Input: part model. Units: mm. Frame: model coordinates. A direction names the side the tool comes from. Give positions to 0.01 mm unless a question says otherwise; leave off trailing zeros. Loops run counter-clockwise (first coordinate to the right, second up) from the corner with the lowest first, then second, coordinate; pieces in that order, holes last.
from build123d import *

# Parameters (mm, degrees)
SKETCH_1_W          = 45.22
SKETCH_1_H          = 24.72
SKETCH_1_R          = 9.6
SKETCH_1_R_2        = 1
EXTRUDE_1_DEPTH     = 3
SKETCH_2_W          = 3
SKETCH_2_H          = 24.72
EXTRUDE_2_DEPTH     = 10
SKETCH_3_W          = 24.72
SKETCH_3_H          = 3
EXTRUDE_3_DEPTH     = 45.22
SKETCH_4_R          = 9.6
SKETCH_4_R_2        = 1
CUT_EXTRUDE_1_DEPTH = 4
FILLET_3_R          = 10
FILLET_4_R          = 5
FILLET_5_R          = 5
FILLET_6_R          = 5
FILLET_7_R          = 5


with BuildPart() as part:
    # 草图1 → 凸台-拉伸1 (new body)
    with BuildSketch(Plane.XY):
        with Locations((21.400674487, -11.617565982)):
            Rectangle(SKETCH_1_W, SKETCH_1_H)
        with Locations((33.900674487, -11.617565982)):
            Circle(SKETCH_1_R, mode=Mode.SUBTRACT)
        with Locations((25.600674487, -1.257565982)):
            Circle(SKETCH_1_R_2, mode=Mode.SUBTRACT)
        with Locations((4.900674487, -1.257565982)):
            Circle(SKETCH_1_R_2, mode=Mode.SUBTRACT)
        with Locations((4.900674487, -21.977565982)):
            Circle(SKETCH_1_R_2, mode=Mode.SUBTRACT)
        with Locations((25.600674487, -21.977565982)):
            Circle(SKETCH_1_R_2, mode=Mode.SUBTRACT)
    extrude(amount=EXTRUDE_1_DEPTH)

    # 草图2 → 凸台-拉伸2 (add)
    with BuildSketch(Plane.ZY.offset(1.209325513)):
        with Locations((1.5, -11.617565982)):
            Rectangle(SKETCH_2_W, SKETCH_2_H)
    extrude(amount=EXTRUDE_2_DEPTH)

    # 草图3 → 凸台-拉伸3 (add)
    with BuildSketch(Plane(origin=(0, 0.742434018, 0), x_dir=(1, 0, 0), z_dir=(0, 1, 0))):
        with Locations((1.150674487, -1.5)):
            Rectangle(SKETCH_3_W, SKETCH_3_H)
    extrude(amount=EXTRUDE_3_DEPTH)

    # 草图4 → 切除-拉伸1 (cut)
    with BuildSketch(Plane.XY.offset(3)):
        with Locations((1.150674487, 35.852434018)):
            Circle(SKETCH_4_R)
        with Locations((-9.209325513, 27.552434018)):
            Circle(SKETCH_4_R_2)
        with Locations((11.510674487, 27.552434018)):
            Circle(SKETCH_4_R_2)
        with Locations((11.510674487, 6.852434018)):
            Circle(SKETCH_4_R_2)
        with Locations((-9.209325513, 6.852434018)):
            Circle(SKETCH_4_R_2)
    extrude(amount=-CUT_EXTRUDE_1_DEPTH, mode=Mode.SUBTRACT)

    # 圆角3
    fillet_3_edges = [part.edges().sort_by_distance(p)[0] for p in [
        (-11.209325513, -23.977565982, 1.5),
    ]]
    fillet(fillet_3_edges, radius=FILLET_3_R)

    # 圆角4
    fillet_4_edges = [part.edges().sort_by_distance(p)[0] for p in [
        (44.010674487, -23.977565982, 1.5),
    ]]
    fillet(fillet_4_edges, radius=FILLET_4_R)

    # 圆角5
    fillet_5_edges = [part.edges().sort_by_distance(p)[0] for p in [
        (44.010674487, 0.742434018, 1.5),
    ]]
    fillet(fillet_5_edges, radius=FILLET_5_R)

    # 圆角6
    fillet_6_edges = [part.edges().sort_by_distance(p)[0] for p in [
        (-11.209325513, 45.962434018, 1.5),
    ]]
    fillet(fillet_6_edges, radius=FILLET_6_R)

    # 圆角7
    fillet_7_edges = [part.edges().sort_by_distance(p)[0] for p in [
        (13.510674487, 45.962434018, 1.5),
    ]]
    fillet(fillet_7_edges, radius=FILLET_7_R)


solid = part.part
(1) Cut plane A-A (y = -17). Return the cut outline in (x, z), and give its area (3 significant figures).
Values follow:
outline: (-10.74, 0) - (25.95, 0) - (25.95, 3) - (-10.74, 3) - close; (41.85, 0) - (44.01, 0) - (44.01, 3) - (41.85, 3) - close
area: 117 mm2
(2) Ray query, probe 1 along Y at (x, z) = (11, 1.4); probe 2 along X at (y, z) = (28, 0.6); probe 3 along Y at (x, z) = (5, 1.45). Return the intervals inside material, ascending.
Values follow:
probe 1: y = -23.98 to 5.99, 7.71 to 26.69, 28.41 to 45.3
probe 2: x = -11.21 to -10.1, -8.32 to -4.37, 6.67 to 10.62, 12.4 to 13.51
probe 3: y = -23.98 to -22.97, -20.98 to -2.25, -0.26 to 27.06, 44.65 to 45.96
(3) Mould query, pull axis X, two halves, no side actions, for faces 3 (the cylindrical face through (10.72, 6.24, 1.52)), 4 (the cylindrical face through (12.007, 44.537, 1.479)), 5 (the cylindrical face through (3.9, -1.21, 1.48)), 6 (the cylindrical face through (-9.706, 44.537, 1.479)). Classes: +X half, -X half, draft (parallel to the pull), parting line (faces both ways), or undercut.
Values follow:
face 3: undercut
face 4: +X half
face 5: undercut
face 6: -X half
(4) Cut plane B-B (x = -2). Return the cut outline in (y, z), and give its area (3 significant figures).
Values follow:
outline: (-23.95, 0) - (26.78, 0) - (26.78, 3) - (-23.95, 3) - close; (44.92, 0) - (45.96, 0) - (45.96, 3) - (44.92, 3) - close
area: 155 mm2
(5) Cut plane D-D (x = 5). Return the cut outline in (y, z).
Values follow:
outline: (-23.98, 0) - (-22.97, 0) - (-22.97, 3) - (-23.98, 3) - close; (-20.98, 0) - (-2.25, 0) - (-2.25, 3) - (-20.98, 3) - close; (-0.26, 0) - (27.06, 0) - (27.06, 3) - (-0.26, 3) - close; (44.65, 0) - (45.96, 0) - (45.96, 3) - (44.65, 3) - close
(6) Cut plane C-C (z = 2.25). Count the separate pieces of the cut face and the enclosed holes in it, and give its area (3 significant figures).
Values follow:
separate pieces: 1
enclosed holes: 10
area: 1,840 mm2
(7) Pin query (flat end, axial travel): pin 1 Ø1.5 at (y, z) = (30.5, 2) entering from +X; pin 2 Ø2.5 at (x, y) = (25.6, -21.98) entering from +Z. Return the tip coordinate at first contact, or that it passes through.
Values follow:
pin 1: stops at x = 13.51
pin 2: stops at z = 3
(8) Reachability of faces 1 (the flat face through (13.511, 21, 2)), 2 (the cylindrical face through (26.554, -0.957, 1.479)) from +Z, -Z, +X, -X, +Y, -Y: full face, straight path, thin tool, end or side. Return the list, or none.
Values follow:
face 1: +Z, -Z, +X, +Y
face 2: +Z, -Z
